from build123d import *

# Parameters (mm, degrees)
SKETCH_R     = 2.7
PAD_DEPTH    = 11
SKETCH001_R  = 11
POCKET_DEPTH = 9


with BuildPart() as part:
    # Sketch → Pad (new body)
    with BuildSketch(Plane.XY):
        with BuildLine():
            Line((20, 39), (0, 39))
            Line((0, 39), (0, 0))
            Line((0, 0), (0, -27.7))
            Line((0, -27.7), (20, -27.7))
            ThreePointArc((20, -27.7), (25.444722, -25.444722), (27.7, -20))
            Line((27.7, 0), (27.7, -20))
            Line((27.7, 31.3), (27.7, 0))
            ThreePointArc((27.7, 31.3), (25.444722, 36.744722), (20, 39))
        make_face()
        with Locations((20, 20)):
            Circle(SKETCH_R, mode=Mode.SUBTRACT)
        with Locations((20, -20)):
            Circle(SKETCH_R, mode=Mode.SUBTRACT)
    pad = extrude(amount=PAD_DEPTH)

    # Mirrored: Pad across Sketch V_Axis
    add(pad.mirror(Plane(origin=(0, 0, 0), x_dir=(0, 0, 1), z_dir=(1, 0, 0))))

    # Sketch001 → Pocket (cut)
    with BuildSketch(Plane.XY):
        with Locations((0, 20)):
            Circle(SKETCH001_R)
    extrude(amount=POCKET_DEPTH, mode=Mode.SUBTRACT)


solid = part.part
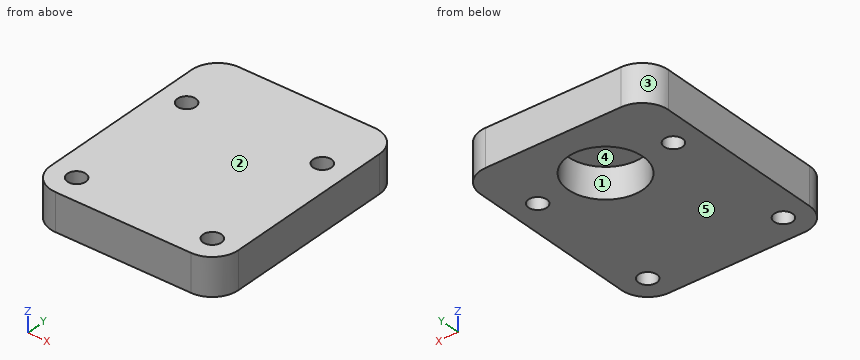
CAD build for the part. Positions are in the model's coordinates, mm. Face numbers are marked on the shaded views. A direction names the side the tool comes from. Round coordinates to 2 decimals unless told otherwise and drop trailing zeros. Loops run counter-clockwise (first coordinate to the right, second up) from the corner with the lowest first, then second, coordinate; pieces in that order, holes last.
(1) Two-plate mould, pull along X, no slides. Class the marked faces 3, 4 and 5: +X half, -X half, draft (parallel to the pull), parting line (faces both ways), or undercut.
(2) Cut at B-B (z = 3.75). Give the cut face in (x, y), plus the area to 3 significant figures.
(3) Cut at A-A (y = 20). Give the cut face in (x, z).
(4) Which spindle directions (+Z, -Z, +X, -X, +Y, -Y) get a long thin tool onto all of the face, cutting with end or side? Do the marked faces 1 and 2. Say none if no direction does.
(5) Cut at C-C (x = 19). Give the cut face in (y, z), plus the area to 3 significant figures.
(6) Cut at D-D (x = -9). Give the cut face in (y, z), plus the area to 3 significant figures.
(7) Wall check: line 1 along Y through (x, z) = (-20, 2.75); line 2 along Y through (x, z) = (0, 2.5); line 3 along Y through (x, z) = (18.5, 5.25) (3 decimals). Give the ranges that are in metal, low to high.
Findings below:
1. face 3: -X half
1. face 4: undercut
1. face 5: draft
2. outline: (-27.7, -20) arc R7.7 ccw to (-20, -27.7) - (20, -27.7) arc R7.7 ccw to (27.7, -20) - (27.7, 31.3) arc R7.7 ccw to (20, 39) - (-20, 39) arc R7.7 ccw to (-27.7, 31.3) - close; hole circle Ø5.4 at (-20, -20); hole circle Ø5.4 at (-20, 20); hole circle Ø22 at (0, 20); hole circle Ø5.4 at (20, -20); hole circle Ø5.4 at (20, 20)
2. area: 3,170 mm2
3. outline: (-27.7, 0) - (-22.7, 0) - (-22.7, 11) - (-27.7, 11) - close; (-17.3, 0) - (-11, 0) - (-11, 9) - (11, 9) - (11, 0) - (17.3, 0) - (17.3, 11) - (-17.3, 11) - close; (22.7, 0) - (27.7, 0) - (27.7, 11) - (22.7, 11) - close
4. face 1: -Z
4. face 2: +Z, +X, -X, +Y, -Y
5. outline: (-27.7, 0) - (-22.51, 0) - (-22.51, 11) - (-27.7, 11) - close; (-17.49, 0) - (17.49, 0) - (17.49, 11) - (-17.49, 11) - close; (22.51, 0) - (39, 0) - (39, 11) - (22.51, 11) - close
5. area: 623 mm2
6. outline: (-27.7, 0) - (13.68, 0) - (13.68, 9) - (26.32, 9) - (26.32, 0) - (39, 0) - (39, 11) - (-27.7, 11) - close
6. area: 620 mm2
7. line 1: y = -27.7 to -22.7, -17.3 to 17.3, 22.7 to 39
7. line 2: y = -27.7 to 9, 31 to 39
7. line 3: y = -27.7 to -22.245, -17.755 to 17.755, 22.245 to 39
